from build123d import *

# Parameters (mm, degrees)
F1_DEPTH = 7
F2_W     = 11
F2_H     = 2
F3_DEPTH = 6.501
F4_R     = 0.99999


# Not quite as in the source:
# - a fillet or chamfer is up to 0.001 mm smaller than in the source, because OpenCascade refuses the exact size


with BuildPart() as f1:
    # F0 (on Top) → F1 (new body)
    with BuildSketch(Plane.XY):
        with BuildLine():
            Line((-2.0766559657, 0), (0, 0))
            Line((0, 0), (13, 0))
            Line((13, 0), (15.0766559657, 0))
            ThreePointArc((15.0766559657, 0), (14.1039701083, 0.5567548152), (13, 0.75))
            Line((13, 0.75), (0, 0.75))
            ThreePointArc((0, 0.75), (-1.1039701083, 0.5567548152), (-2.0766559657, 0))
        make_face()
        with BuildLine():
            ThreePointArc((-2.5, -2.5), (-1.767766953, -0.732233047), (0, 0))
            Line((0, 0), (-2.0766559657, 0))
            ThreePointArc((-2.0766559657, 0), (-2.2980970389, -0.2019029611), (-2.5, -0.4233440343))
            Line((-2.5, -0.4233440343), (-2.5, -2.5))
        make_face()
        with BuildLine():
            ThreePointArc((0, -5), (-1.767766953, -4.267766953), (-2.5, -2.5))
            Line((-2.5, -2.5), (-2.5, -4.5766559657))
            ThreePointArc((-2.5, -4.5766559657), (-2.2980970389, -4.7980970389), (-2.0766559657, -5))
            Line((-2.0766559657, -5), (0, -5))
        make_face()
        with BuildLine():
            Line((-2.5, -4.5766559657), (-2.5, -2.5))
            Line((-2.5, -2.5), (-2.5, -0.4233440343))
            ThreePointArc((-2.5, -0.4233440343), (-3.25, -2.5), (-2.5, -4.5766559657))
        make_face()
        with BuildLine():
            Line((15.5, -0.4233440343), (15.5, -2.5))
            Line((15.5, -2.5), (15.5, -4.5766559657))
            ThreePointArc((15.5, -4.5766559657), (16.25, -2.5), (15.5, -0.4233440343))
        make_face()
        with BuildLine():
            Line((15.0766559657, 0), (13, 0))
            ThreePointArc((13, 0), (14.767766953, -0.732233047), (15.5, -2.5))
            Line((15.5, -2.5), (15.5, -0.4233440343))
            ThreePointArc((15.5, -0.4233440343), (15.2980970389, -0.2019029611), (15.0766559657, 0))
        make_face()
        with BuildLine():
            Line((15.5, -4.5766559657), (15.5, -2.5))
            ThreePointArc((15.5, -2.5), (14.767766953, -4.267766953), (13, -5))
            Line((13, -5), (15.0766559657, -5))
            ThreePointArc((15.0766559657, -5), (15.2980970389, -4.7980970389), (15.5, -4.5766559657))
        make_face()
        with BuildLine():
            Line((13, -5), (0, -5))
            Line((0, -5), (-2.0766559657, -5))
            ThreePointArc((-2.0766559657, -5), (-1.1039701083, -5.5567548152), (0, -5.75))
            Line((0, -5.75), (13, -5.75))
            ThreePointArc((13, -5.75), (14.1039701083, -5.5567548152), (15.0766559657, -5))
            Line((15.0766559657, -5), (13, -5))
        make_face()
    extrude(amount=F1_DEPTH)

    # F2 (on face) → F3 (cut, through all)
    with BuildSketch(Plane.XZ.offset(5.75)):
        with Locations((6.5, 3.5)):
            Rectangle(F2_W, F2_H)
    extrude(amount=-F3_DEPTH, mode=Mode.SUBTRACT)

    # F4 (radius 1 in the source; OpenCascade refuses exactly that, so slightly less here)
    f4_edges = [f1.edges().sort_by_distance(p)[0] for p in [
        (1, -5.375, 4.5),
        (1, -5.375, 2.5),
        (12, -5.375, 2.5),
        (12, 0.375, 4.5),
        (12, -5.375, 4.5),
        (12, 0.375, 2.5),
        (1, 0.375, 2.5),
        (1, 0.375, 4.5),
    ]]
    fillet(f4_edges, radius=F4_R)


solid = f1.part
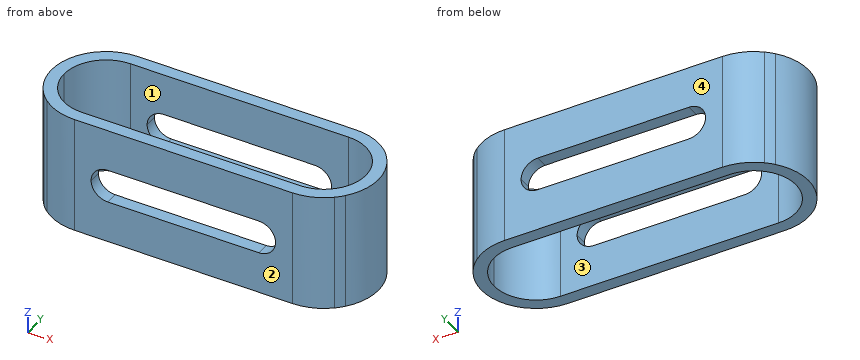
For this review, take the finished solid that the model builds, in its own axes (mm). Face numbers are marked on the shaded views. A direction names the side the tool comes from. Give positions to 0.01 mm unless a question says otherwise; leave off trailing zeros. Loops run counter-clockwise (first coordinate to the right, second up) from the corner with the lowest first, then second, coordinate; pieces in that order, holes last. Notation, with made-up numbers: M 27.25,6 L 42.25,6 A19 ccw 42.25,19 Z; hole C 38,-11.75 d1. An arc over 180 degrees is marked long. Put each result on its own line as item: value. Start each with the question number.
(1) Add section B-B, the plane z = 6. Write out the cut boundary in (x, y).
(2) Machinability: for the marked faces 1 and 2, which of the approach directions +Z, -Z, +X, -X, +Y, -Y give a long, thin tool a straight path to every point of the face, cutting with its end or side? Answer none if there is none.
(3) Add section D-D, the plane x = 7.75. Write out the cut boundary in (y, z).
(4) Add section C-C, the plane y = -0.75. Write out the cut boundary in (x, z).
(5) Add section A-A, the plane x = 0.75. Write out the cut boundary in (y, z).
(6) The part is to be moulded in two halves that separate along X. For the marked faces 3 and 4, say which applies: +X half, -X half, draft (parallel to the pull), parting line (faces both ways), or undercut.
(7) Wall thickness on L1, parallel to Y at x = 3, z = 6.75; L2, parallel to X at y = -3.75, z = 3.25; L3, parallel to X at y = -1.5, z = 4.25: over which ranges is each line inside the solid? List them lowest first.
Result:
1. outline: M 0,-5.75 L 13,-5.75 A3.25 ccw 13,0.75 L 0,0.75 A3.25 ccw Z; hole M 0,-5 L 13,-5 A2.5 ccw 13,0 L 0,0 A2.5 ccw Z
2. face 1: +Z, -Z
2. face 2: +Z, -Z, +X, -X, -Y
3. outline: M -5.75,0 L -5,0 L -5,2.5 L -5.75,2.5 Z; M -5.75,4.5 L -5,4.5 L -5,7 L -5.75,7 Z; M 0,0 L 0.75,0 L 0.75,2.5 L 0,2.5 Z; M 0,4.5 L 0.75,4.5 L 0.75,7 L 0,7 Z
4. outline: M -2.74,0 L -1.79,0 L -1.79,7 L -2.74,7 Z; M 14.79,0 L 15.74,0 L 15.74,7 L 14.79,7 Z
5. outline: M -5.75,0 L -5,0 L -5,7 L -5.75,7 Z; M 0,0 L 0.75,0 L 0.75,7 L 0,7 Z
6. face 3: undercut
6. face 4: draft
7. L1: y = -5.75 to -5, 0 to 0.75
7. L2: x = -3 to -2.17, 15.17 to 16
7. L3: x = -3.09 to -2.29, 15.29 to 16.09
